from build123d import *

# Parameters (mm, degrees)
F0_R     = 4.75
F0_R_2   = 2.55
F1_DEPTH = 3
F2_R     = 2.5
F3_SIZE  = 0.2


with BuildPart() as f1:
    # F0 (on Top) → F1 (new body)
    with BuildSketch(Plane.XY):
        Polygon((-42.4056542814, 90), (-42.4056542814, 0), (67.5943457186, 0), (67.5943457186, 90), (57.5943457186, 100), (37.5943457186, 100), (37.5943457186, 90), (-12.4056542814, 90), (-12.4056542814, 100), (-32.4056542814, 100), align=None)
        with Locations((-31.1556542814, 19)):
            Circle(F0_R, mode=Mode.SUBTRACT)
        with Locations((-18.6556542814, 19)):
            Circle(F0_R, mode=Mode.SUBTRACT)
        with Locations((-6.1556542814, 19)):
            Circle(F0_R, mode=Mode.SUBTRACT)
        with Locations((6.3443457186, 19)):
            Circle(F0_R, mode=Mode.SUBTRACT)
        with Locations((-31.1556542814, 31.5)):
            Circle(F0_R, mode=Mode.SUBTRACT)
        with Locations((-18.6556542814, 31.5)):
            Circle(F0_R, mode=Mode.SUBTRACT)
        with Locations((-31.1556542814, 44)):
            Circle(F0_R, mode=Mode.SUBTRACT)
        with Locations((-18.6556542814, 44)):
            Circle(F0_R, mode=Mode.SUBTRACT)
        with Locations((-6.1556542814, 31.5)):
            Circle(F0_R, mode=Mode.SUBTRACT)
        with Locations((6.3443457186, 31.5)):
            Circle(F0_R, mode=Mode.SUBTRACT)
        with Locations((-6.1556542814, 44)):
            Circle(F0_R, mode=Mode.SUBTRACT)
        with Locations((6.3443457186, 44)):
            Circle(F0_R, mode=Mode.SUBTRACT)
        with Locations((27.5943457186, 6)):
            Circle(F0_R_2, mode=Mode.SUBTRACT)
        with Locations((18.8443457186, 19)):
            Circle(F0_R, mode=Mode.SUBTRACT)
        with Locations((31.3443457186, 19)):
            Circle(F0_R, mode=Mode.SUBTRACT)
        with Locations((43.8443457186, 19)):
            Circle(F0_R, mode=Mode.SUBTRACT)
        with Locations((56.3443457186, 19)):
            Circle(F0_R, mode=Mode.SUBTRACT)
        with Locations((18.8443457186, 31.5)):
            Circle(F0_R, mode=Mode.SUBTRACT)
        with Locations((31.3443457186, 31.5)):
            Circle(F0_R, mode=Mode.SUBTRACT)
        with Locations((18.8443457186, 44)):
            Circle(F0_R, mode=Mode.SUBTRACT)
        with Locations((31.3443457186, 44)):
            Circle(F0_R, mode=Mode.SUBTRACT)
        with Locations((43.8443457186, 31.5)):
            Circle(F0_R, mode=Mode.SUBTRACT)
        with Locations((56.3443457186, 31.5)):
            Circle(F0_R, mode=Mode.SUBTRACT)
        with Locations((43.8443457186, 44)):
            Circle(F0_R, mode=Mode.SUBTRACT)
        with Locations((56.3443457186, 44)):
            Circle(F0_R, mode=Mode.SUBTRACT)
        with Locations((-31.1556542814, 56.5)):
            Circle(F0_R, mode=Mode.SUBTRACT)
        with Locations((-18.6556542814, 56.5)):
            Circle(F0_R, mode=Mode.SUBTRACT)
        with Locations((-31.1556542814, 69)):
            Circle(F0_R, mode=Mode.SUBTRACT)
        with Locations((-18.6556542814, 69)):
            Circle(F0_R, mode=Mode.SUBTRACT)
        with Locations((-6.1556542814, 56.5)):
            Circle(F0_R, mode=Mode.SUBTRACT)
        with Locations((6.3443457186, 56.5)):
            Circle(F0_R, mode=Mode.SUBTRACT)
        with Locations((-6.1556542814, 69)):
            Circle(F0_R, mode=Mode.SUBTRACT)
        with Locations((6.3443457186, 69)):
            Circle(F0_R, mode=Mode.SUBTRACT)
        with Locations((-31.1556542814, 81.5)):
            Circle(F0_R, mode=Mode.SUBTRACT)
        with Locations((-18.6556542814, 81.5)):
            Circle(F0_R, mode=Mode.SUBTRACT)
        with Locations((-22.4056542814, 94)):
            Circle(F0_R_2, mode=Mode.SUBTRACT)
        with Locations((-6.1556542814, 81.5)):
            Circle(F0_R, mode=Mode.SUBTRACT)
        with Locations((6.3443457186, 81.5)):
            Circle(F0_R, mode=Mode.SUBTRACT)
        with Locations((18.8443457186, 56.5)):
            Circle(F0_R, mode=Mode.SUBTRACT)
        with Locations((31.3443457186, 56.5)):
            Circle(F0_R, mode=Mode.SUBTRACT)
        with Locations((18.8443457186, 69)):
            Circle(F0_R, mode=Mode.SUBTRACT)
        with Locations((31.3443457186, 69)):
            Circle(F0_R, mode=Mode.SUBTRACT)
        with Locations((43.8443457186, 56.5)):
            Circle(F0_R, mode=Mode.SUBTRACT)
        with Locations((56.3443457186, 56.5)):
            Circle(F0_R, mode=Mode.SUBTRACT)
        with Locations((43.8443457186, 69)):
            Circle(F0_R, mode=Mode.SUBTRACT)
        with Locations((56.3443457186, 69)):
            Circle(F0_R, mode=Mode.SUBTRACT)
        with Locations((18.8443457186, 81.5)):
            Circle(F0_R, mode=Mode.SUBTRACT)
        with Locations((31.3443457186, 81.5)):
            Circle(F0_R, mode=Mode.SUBTRACT)
        with Locations((43.8443457186, 81.5)):
            Circle(F0_R, mode=Mode.SUBTRACT)
        with Locations((56.3443457186, 81.5)):
            Circle(F0_R, mode=Mode.SUBTRACT)
        with Locations((47.5943457186, 94)):
            Circle(F0_R_2, mode=Mode.SUBTRACT)
    extrude(amount=F1_DEPTH)

    # F2
    f2_edges = [f1.edges().sort_by_distance(p)[0] for p in [
        (-12.405654, 90, 1.5),
        (37.594346, 90, 1.5),
    ]]
    fillet(f2_edges, radius=F2_R)

    # F3
    f3_edges = [f1.edges().sort_by_distance(p)[0] for p in [
        (12.594346, 0, 0),
        (67.594346, 45, 0),
        (-42.405654, 45, 0),
        (62.594346, 95, 0),
        (47.594346, 100, 0),
        (-12.405654, 96.25, 0),
        (-22.405654, 100, 0),
        (-37.405654, 95, 0),
        (-11.673421, 90.732233, 0),
        (36.862113, 90.732233, 0),
        (37.594346, 96.25, 0),
        (12.594346, 90, 0),
    ]]
    chamfer(f3_edges, length=F3_SIZE)


solid = f1.part
Geometry: final body of the model. Coordinates: model frame, mm. Give positions to 0.01 mm unless a question says otherwise; leave off trailing zeros. Write each loop counter-clockwise with the first axis right and the second up, starting at its lowest first coordinate (ties: lowest second). Pieces come first, ordered by that corner, then holes. Notation, with made-up numbers: (33.25, -30.5) - (58.25, -30.5) arc R9 cw to (58.25, -17.5) - close; hole circle Ø10 at (9.5, 33). An arc over 180 degrees is marked (long way). Return JSON: item names as keys, results as strings. Group by question number.
1) Section B-B on y = 94. Return the cut outline in (x, z), plus the area to 3 significant figures.
2) Mould query, pull axis X, two halves, no side actions, for faces 1 (the flat face through (12, 0, 2)), 2 (the flat face through (67.594, 44, 2)), 3 (the cylindrical face through (5.315, 51.863, 1.479)). Classes: released by +X, released by -X, zero draft, split by the parting line, or undercut.
3) Section A-A on x = -7. State how many separate pieces and enclosed holes the cut face has, plus the area to 3 significant figures.
4) Line query: line 1 (X direction, y = 95, z = 1.45); line 2 (Y direction, x = -11.5, z = 1). Output: solid intervals per line, ascending.
Filled in:
{
 "1": {"outline": "(-38.41, 0.2) - (-38.12, 0) - (-24.96, 0) - (-24.96, 3) - (-38.41, 3) - close; (-19.86, 0) - (-12.61, 0) - (-12.41, 0.2) - (-12.41, 3) - (-19.86, 3) - close; (37.59, 0.2) - (37.79, 0) - (45.04, 0) - (45.04, 3) - (37.59, 3) - close; (50.14, 0) - (63.31, 0) - (63.59, 0.2) - (63.59, 3) - (50.14, 3) - close", "area": "125 mm^2"},
 "2": {"face 1": "zero draft", "face 2": "released by +X", "face 3": "undercut"},
 "3": {"separate pieces": "7", "enclosed holes": "0", "area": "102 mm^2"},
 "4": {"line 1": "x = -37.41 to -24.75, -20.06 to -12.41, 37.59 to 45.25, 49.94 to 62.59", "line 2": "y = 0 to 90.57"}
}
